```python
from build123d import *

# Parameters (mm, degrees)
ESBO_O1_W                = 110
ESBO_O1_H                = 150
RESSALTO_EXTRUS_O3_DEPTH = 8
FILETE2_R                = 5
CASCA1_T                 = -3
RESSALTO_EXTRUS_O7_START = 5
ESBO_O14_R               = 5
RESSALTO_EXTRUS_O7_DEPTH = 5
RESSALTO_EXTRUS_O4_START = -8
RESSALTO_EXTRUS_O4_DEPTH = 5
FILETE6_R                = 2
FILETE8_R                = 5
ESBO_O15_R               = 1.7
CORTE_EXTRUS_O3_DEPTH    = 3
ESBO_O18_R               = 5.25
CORTE_EXTRUS_O7_DEPTH    = 5
ESBO_O19_W               = 72.5
ESBO_O19_H               = 27.5
CORTE_EXTRUS_O8_DEPTH    = 5
FILETE9_R                = 3
FILETE10_R               = 1
ESBO_O20_R               = 3
CORTE_EXTRUS_O9_DEPTH    = 10
ESBO_O22_W               = 13.52
ESBO_O22_H               = 9.06512497
CORTE_EXTRUS_O11_DEPTH   = 20
ESBO_O8_W                = 3
ESBO_O8_H                = 13.5
RESSALTO_EXTRUS_O9_DEPTH = 1


with BuildPart() as part:
    # Esboço1 → Ressalto-extrusão3 (new body)
    with BuildSketch(Plane(origin=(0, 0, 0), x_dir=(1, 0, 0), z_dir=(0, 1, 0))):
        Rectangle(ESBO_O1_W, ESBO_O1_H)
    extrude(amount=-RESSALTO_EXTRUS_O3_DEPTH)

    # Filete2
    filete2_edges = [part.edges().sort_by_distance(p)[0] for p in [
        (55, -4, 75),
        (-55, -4, 75),
        (-55, -4, -75),
        (55, -4, -75),
    ]]
    fillet(filete2_edges, radius=FILETE2_R)

    # Casca1
    casca1_openings = [part.faces().sort_by_distance(p)[0] for p in [
        (0, -8, 0),
    ]]
    offset(amount=CASCA1_T, openings=casca1_openings, kind=Kind.INTERSECTION)

    # Esboço14 → Ressalto-extrusão7 (add)
    with BuildSketch(Plane(origin=(0, -3, 0), x_dir=(-1, 0, 0), z_dir=(0, -1, 0)).offset(RESSALTO_EXTRUS_O7_START)):
        with Locations((50, -70)):
            Circle(ESBO_O14_R)
        with Locations((-50, -70)):
            Circle(ESBO_O14_R)
        with Locations((-50, 70)):
            Circle(ESBO_O14_R)
        with Locations((50, 70)):
            Circle(ESBO_O14_R)
    extrude(amount=-RESSALTO_EXTRUS_O7_DEPTH)

    # Esboço6 → Ressalto-extrusão4 (add)
    with BuildSketch(Plane(origin=(0, 0, 0), x_dir=(1, 0, 0), z_dir=(0, 1, 0)).offset(RESSALTO_EXTRUS_O4_START)):
        Polygon((-32, -37), (32, -37), (32, -72), (35, -72), (35, -34), (-35, -34), (-35, -72), (-32, -72), align=None)
    extrude(amount=RESSALTO_EXTRUS_O4_DEPTH)

    # Filete6
    filete6_edges = [part.edges().sort_by_distance(p)[0] for p in [
        (-32, -5.5, 72),
        (-32, -5.5, 37),
        (32, -5.5, 37),
        (32, -5.5, 72),
    ]]
    fillet(filete6_edges, radius=FILETE6_R)

    # Filete8
    filete8_edges = [part.edges().sort_by_distance(p)[0] for p in [
        (35, -5.5, 34),
        (-35, -5.5, 34),
        (-35, -5.5, 72),
        (35, -5.5, 72),
    ]]
    fillet(filete8_edges, radius=FILETE8_R)

    # Esboço15 → Corte-extrusão3 (cut)
    with BuildSketch(Plane.XZ.offset(8)):
        with Locations(Location((-50, -70, 0), (0, 0, 270))):
            Circle(ESBO_O15_R)
        with Locations(Location((50, -70, 0), (0, 0, 270))):
            Circle(ESBO_O15_R)
        with Locations(Location((50, 70, 0), (0, 0, 270))):
            Circle(ESBO_O15_R)
        with Locations(Location((-50, 70, 0), (0, 0, 270))):
            Circle(ESBO_O15_R)
    extrude(amount=-CORTE_EXTRUS_O3_DEPTH, mode=Mode.SUBTRACT)

    # Esboço18 → Corte-extrusão7 (cut)
    with BuildSketch(Plane(origin=(0, 0, 0), x_dir=(1, 0, 0), z_dir=(0, 1, 0))):
        with Locations(Location((-34, 10.1, 0), (0, 0, 270))):
            Circle(ESBO_O18_R)
        with Locations(Location((-11.333333333, 10.1, 0), (0, 0, 270))):
            Circle(ESBO_O18_R)
        with Locations(Location((11.333333333, 10.1, 0), (0, 0, 270))):
            Circle(ESBO_O18_R)
        with Locations(Location((34, 10.1, 0), (0, 0, 270))):
            Circle(ESBO_O18_R)
    extrude(amount=-CORTE_EXTRUS_O7_DEPTH, mode=Mode.SUBTRACT)

    # Esboço19 → Corte-extrusão8 (cut)
    with BuildSketch(Plane(origin=(0, 0, 0), x_dir=(1, 0, 0), z_dir=(0, 1, 0))):
        with Locations((-0.25, 35.25)):
            Rectangle(ESBO_O19_W, ESBO_O19_H)
    extrude(amount=-CORTE_EXTRUS_O8_DEPTH, mode=Mode.SUBTRACT)

    # Filete9
    filete9_edges = [part.edges().sort_by_distance(p)[0] for p in [
        (36, 0, -35.25),
        (-0.25, 0, -49),
        (-36.5, 0, -35.25),
        (-0.25, 0, -21.5),
    ]]
    fillet(filete9_edges, radius=FILETE9_R - 0.0001)  # a hair under: the kernel refuses the full size

    # Filete10
    filete10_edges = [part.edges().sort_by_distance(p)[0] for p in [
        (-34, 0, -15.35),
        (-11.333333333, 0, -15.35),
        (11.333333333, 0, -15.35),
        (34, 0, -15.35),
    ]]
    fillet(filete10_edges, radius=FILETE10_R)

    # Esboço20 → Corte-extrusão9 (cut)
    with BuildSketch(Plane(origin=(0, 0, 0), x_dir=(1, 0, 0), z_dir=(0, 1, 0))):
        with Locations(Location((12.42, -19.11, 0), (0, 0, 270))):
            Circle(ESBO_O20_R)
        with Locations(Location((20.04, -19.11, 0), (0, 0, 270))):
            Circle(ESBO_O20_R)
    extrude(amount=-CORTE_EXTRUS_O9_DEPTH, mode=Mode.SUBTRACT)

    # Esboço22 → Corte-extrusão11 (cut)
    with BuildSketch(Plane.ZY.offset(55)):
        with Locations((14.11, -7.032562485)):
            Rectangle(ESBO_O22_W, ESBO_O22_H)
    extrude(amount=-CORTE_EXTRUS_O11_DEPTH, mode=Mode.SUBTRACT)

    # Esboço8 → Ressalto-extrusão9 (add)
    with BuildSketch(Plane(origin=(0, -8, 0), x_dir=(-1, 0, 0), z_dir=(0, -1, 0))):
        with Locations((-53.5, -48.25)):
            Rectangle(ESBO_O8_W, ESBO_O8_H)
    extrude(amount=RESSALTO_EXTRUS_O9_DEPTH)


solid = part.part
```
Verification items for the finished model (mm, model axes). A direction names the side the tool comes from. Coordinates: 2 decimals unless noted, no trailing zeros. Write each loop counter-clockwise with the first axis right and the second up, starting at its lowest first coordinate (ties: lowest second). Pieces come first, ordered by that corner, then holes. Notation, with made-up numbers: M -30,13 L 12,13 A27 cw 12,43 Z; hole C -18.75,81 d7. An arc over 180 degrees is marked long. Answer as a JSON object with one key per item and string values. Group by question number.
(1) Tool access check on faces 5 (the face through (-37.4, -0.86, -35.48)), 6 (the face through (50, -5, -70)), 7 (the face through (-50.2, -2.8, 7.35)). Record the directions out of +Z, -Z, +X, -X, +Y, -Y that give a thin tool (end or side, any length) a straight path to the whole face; none if there is none.
(2) Release check for a two-part mould opening along X. For faces 1 (the face through (-54, -4, -73)), 2 (the face through (-43, -5, 72)), 3 (the face through (0, -6, 34)), 4 (the face through (-8, -8, 74)) record: +X half, -X half, draft (parallel to the pull), parting line (faces both ways), or undercut.
(3) Cross-section at C-C, the plane z = 50.5. Record the cut outline in (x, y).
(4) Gauge pin test, flat ends, axial feed: pin 1 (7 mm diameter, centred on x = -49, z = 12, fed in from -Y); pin 2 (6 mm diameter, centred on x = -29, z = -23.5, fed in from -Y); pin 3 (6.5 mm diameter, centred on x = 11.33, z = -10.1, fed in from +Y); pin 4 (0.5 mm diameter, centred on x = 53, y = -8.5, fed in from -Z). Record the tip position at first contact, or that the pin passes through.
(5) Material ranges on line 1 (Z direction, x = -12, y = -5.5); line 2 (X direction, y = -6.75, z = 48.5); line 3 (X direction, y = -0.95, z = 19.11), recorded low to high.
(6) Cross-section at A-A, the plane z = 19.11. Record the cut outline in (x, y), and give its area (3 significant figures).
Reply:
{
 "1": {"face 5": "+Y", "face 6": "-Y", "face 7": "-X, -Y"},
 "2": {"face 1": "-X half", "face 2": "undercut", "face 3": "undercut", "face 4": "draft"},
 "3": {"outline": "M -55,-8 L -52,-8 L -52,-3 L -35,-3 L -35,-8 L -32,-8 L -32,-3 L 32,-3 L 32,-8 L 35,-8 L 35,-3 L 52,-3 L 52,-9 L 55,-9 L 55,0 L -55,0 Z"},
 "4": {"pin 1": "y = -2.5", "pin 2": "y = -3", "pin 3": "through", "pin 4": "z = 41.5"},
 "5": {"line 1": "-75 to -72, 34 to 37, 72 to 75", "line 2": "-55 to -52, -35 to -32, 32 to 35, 52 to 55", "line 3": "-55 to 9.42, 15.42 to 17.04, 23.04 to 55"},
 "6": {"outline": "M -55,-2.5 L -35,-2.5 L -35,-3 L 9.42,-3 L 9.42,0 L -55,0 Z; M 15.42,-3 L 17.04,-3 L 17.04,0 L 15.42,0 Z; M 23.04,-3 L 52,-3 L 52,-8 L 55,-8 L 55,0 L 23.04,0 Z", "area": "299 mm²"}
}
